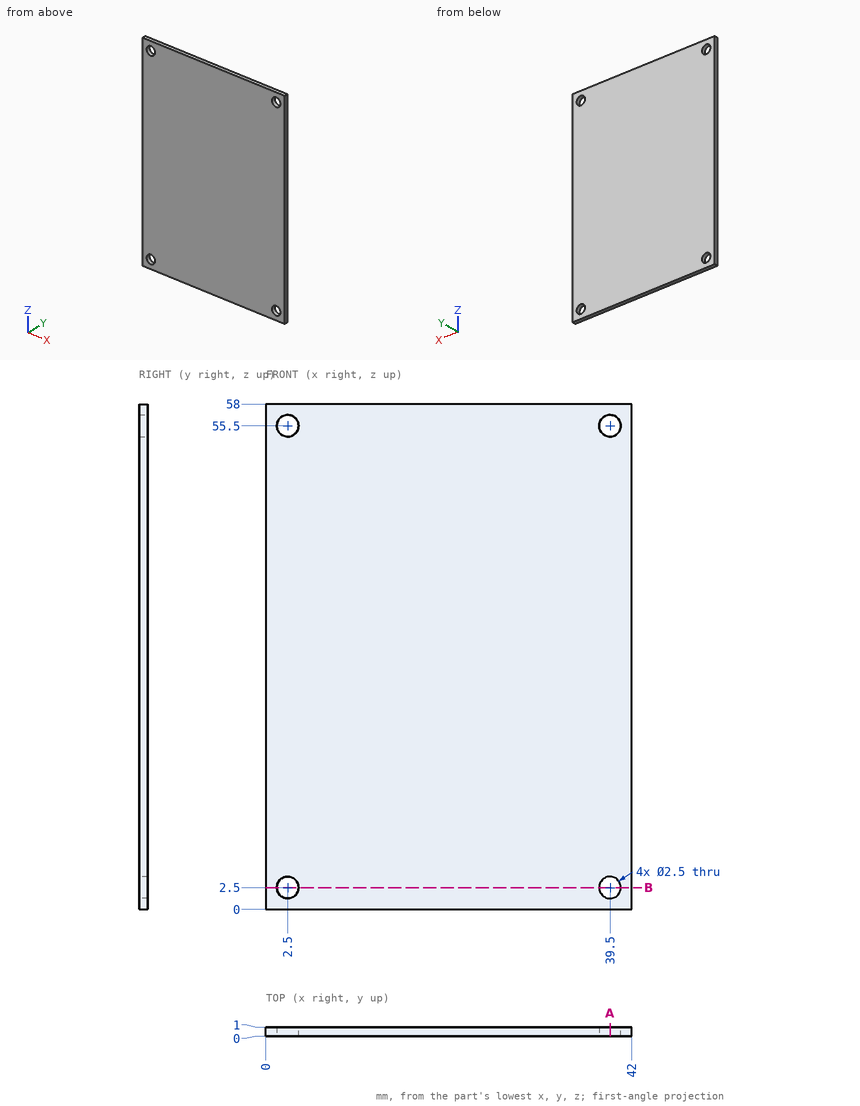
Geometry check sheet. Reference: drawing and pictorial views, mm from the part's lowest x, y, z. Coordinates: 2 decimals unless noted, no trailing zeros. Loops run counter-clockwise (first coordinate to the right, second up) from the corner with the lowest first, then second, coordinate; pieces in that order, holes last. Notation, with made-up numbers: (89.5, -36) -> (104.5, -36) arc R35 cw to (104.5, -2) -> close; hole circle Ø8 at (18, -27). An arc over 180 degrees is marked (long way). Write item = value, one per line. Start each with the question number.
1. Section check B-B on z = 2.5. Record the cut outline in (x, y).
2. Material ranges on line 1 (Z direction, x = 2.5, y = 0.55); line 2 (X direction, y = 0.75, z = 55.5), recorded low to high.
3. Section check A-A on x = 39.5. Record the cut outline in (y, z).
4. Depth check by flat-ended pin: P1, Ø3, axis at x = 39.5, z = 2.5, coming from the +Y side; P2, Ø1.5, axis at x = 39.5, z = 55.5, coming from the +Y side. Enter the tip coordinate at first touch or a pass-through.
Responses:
q1.outline = (0, 0) -> (1.25, 0) -> (1.25, 1) -> (0, 1) -> close; (3.75, 0) -> (38.25, 0) -> (38.25, 1) -> (3.75, 1) -> close; (40.75, 0) -> (42, 0) -> (42, 1) -> (40.75, 1) -> close
q2.line_1 = 0 to 1.25, 3.75 to 54.25, 56.75 to 58
q2.line_2 = 0 to 1.25, 3.75 to 38.25, 40.75 to 42
q3.outline = (0, 0) -> (1, 0) -> (1, 1.25) -> (0, 1.25) -> close; (0, 3.75) -> (1, 3.75) -> (1, 54.25) -> (0, 54.25) -> close; (0, 56.75) -> (1, 56.75) -> (1, 58) -> (0, 58) -> close
q4.P1 = 1
q4.P2 = through
